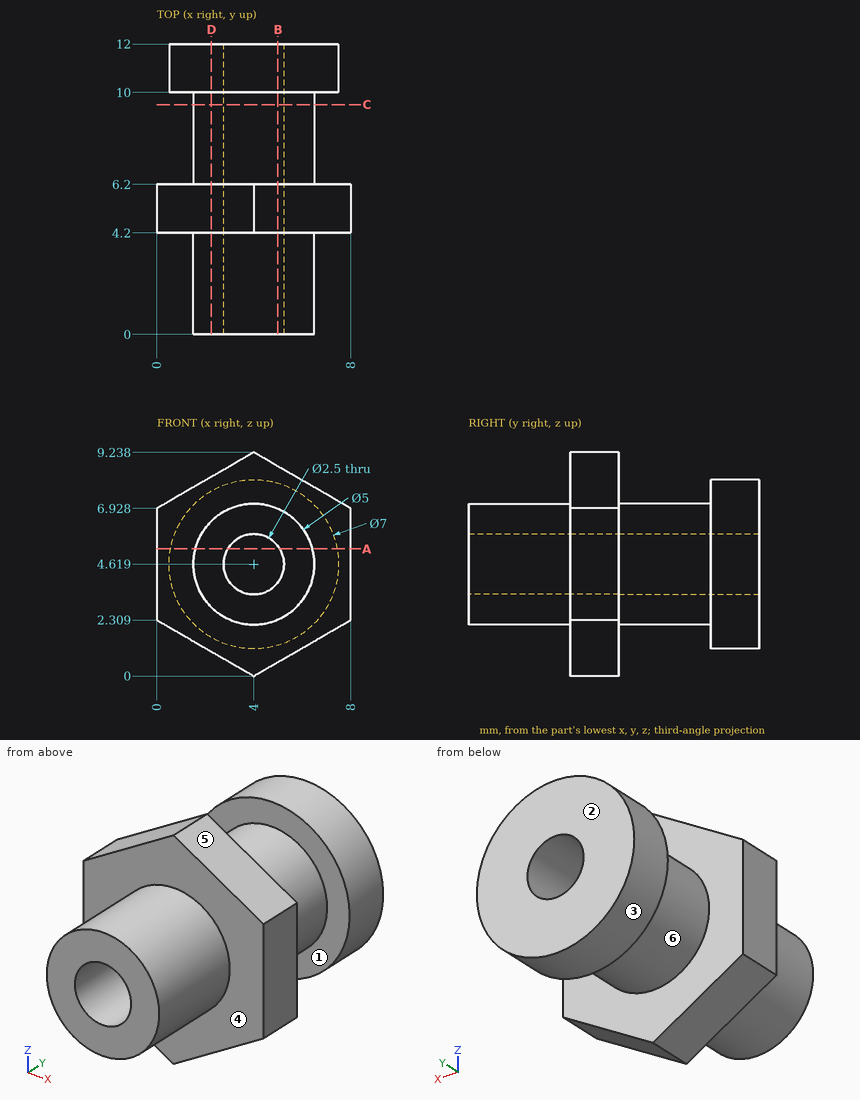
Check sheet for the drawn part. Datum: minimum x, y, z corner. Units: mm. A direction names the side the tool comes from. Round coordinates to 2 decimals unless told otherwise and drop trailing zeros. Order: outer loops, then holes, each group sorted by start corner. A loop starts at its lowest first (then second) coordinate and runs counter-clockwise, first axis right, second up. Notation, with made-up numbers: M -20.75,61.25 L -12.75,61.25 A10 ccw -12.75,70.25 Z; hole C 61,24.25 d6. An arc over 180 degrees is marked long. Write each question's results on one line, items separated by ' | '. Start each with the question number.
1. Cross-section at D-D on x = 2.25. Record the boundary of the cut face in (y, z).
2. Cross-section at B-B on x = 5. Record the boundary of the cut face in (y, z) (1 decimal).
3. Go/stop test with flat-tipped pins: P1, Ø3, axis at x = 4, z = 4.62, coming from the -Y side; P2, Ø2, axis at y = 7.5, z = 4, coming from the +X side. Record where each tip stops, or that it passes through.
4. Set-up check for the marked faces 4, 5 and 6: record each of +Z, -Z, +X, -X, +Y, -Y from which the full face is reachable in a straight line by a thin tool's end or side.
5. Cross-section at C-C on y = 9.5. Record the boundary of the cut face in (x, z).
6. Cross-section at A-A on z = 5.25. Record the boundary of the cut face in (x, y).
7. Draft check along Y on the marked faces 1, 2 and 3. Enter one of: pulls with the +Y half, pulls with the -Y half, needs draft (parallel to the pull), parting line crosses it, or undercut.
8. Material ranges on L1, parallel to Y at x = 4.5, z = 1.5; L2, parallel to Z at x = 4, y = 9.3; L3, parallel to X at y = 2.5, z = 4.25 (1 decimal), recorded low to high. Write a range as from..to.
Resolved:
1) outline: M 0,2.83 L 4.2,2.83 L 4.2,1.01 L 6.2,1.01 L 6.2,2.83 L 10,2.83 L 10,1.59 L 12,1.59 L 12,7.65 L 10,7.65 L 10,6.4 L 6.2,6.4 L 6.2,8.23 L 4.2,8.23 L 4.2,6.4 L 0,6.4 Z
2) outline: M 0,2.3 L 4.2,2.3 L 4.2,0.6 L 6.2,0.6 L 6.2,2.3 L 10,2.3 L 10,1.3 L 12,1.3 L 12,3.9 L 0,3.9 Z; M 0,5.4 L 12,5.4 L 12,8 L 10,8 L 10,6.9 L 6.2,6.9 L 6.2,8.7 L 4.2,8.7 L 4.2,6.9 L 0,6.9 Z
3) P1: y = 0 | P2: x = 6.5
4) face 4: -Y | face 5: +Z, +X, +Y, -Y | face 6: none
5) outline: C 4,4.62 d5; hole C 4,4.62 d2.5
6) outline: M 0,4.2 L 1.58,4.2 L 1.58,0 L 2.92,0 L 2.92,12 L 0.56,12 L 0.56,10 L 1.58,10 L 1.58,6.2 L 0,6.2 Z; M 5.08,0 L 6.42,0 L 6.42,4.2 L 8,4.2 L 8,6.2 L 6.42,6.2 L 6.42,10 L 7.44,10 L 7.44,12 L 5.08,12 Z
7) face 1: undercut | face 2: pulls with the +Y half | face 3: needs draft
8) L1: 4.2..6.2, 10..12 | L2: 2.12..3.37, 5.87..7.12 | L3: 1.5..2.8, 5.2..6.5
